The listing builds one solid part. Answer for the finished solid, in the listing's coordinates (mm). A direction names the side the tool comes from. Round coordinates to 2 decimals unless told otherwise and drop trailing zeros. Loops run counter-clockwise (first coordinate to the right, second up) from the corner with the lowest first, then second, coordinate; pieces in that order, holes last. Notation, with made-up numbers: M -38,76 L -12,76 A21 cw -12,82 Z; hole C 69,-5 d6. An arc over 180 degrees is marked long. Answer as a JSON object with one key per item and string values.
```python
from build123d import *

# Parameters (mm, degrees)
F0_W      = 380
F0_H      = 180
F1_DEPTH  = 10
F2_W      = 6
F2_H      = 180
F3_DEPTH  = 2
F5_DEPTH  = 5.6
F7_DEPTH  = 5.8
F8_R      = 3.5
F9_DEPTH  = 5
F9_TAPER  = 1
F10_R     = 3.5
F11_DEPTH = 5


with BuildPart() as f1:
    # F0 (on Top) → F1 (new body)
    with BuildSketch(Plane.XY):
        Rectangle(F0_W, F0_H)
    extrude(amount=F1_DEPTH)

    # F2 (on face) → F3 (join)
    with BuildSketch(Plane.XY.offset(10)):
        Rectangle(F2_W, F2_H)
    extrude(amount=F3_DEPTH)

    # F4 (on face) → F5 (cut)
    with BuildSketch(Plane.XY.offset(10)):
        with BuildLine():
            ThreePointArc((-4.5, 49), (-6.2573593129, 53.2426406871), (-10.5, 55))
            Line((-10.5, 55), (-139.5, 55))
            ThreePointArc((-139.5, 55), (-143.7426406871, 53.2426406871), (-145.5, 49))
            Line((-145.5, 49), (-145.5, -49))
            ThreePointArc((-145.5, -49), (-143.7426406871, -53.2426406871), (-139.5, -55))
            Line((-139.5, -55), (-10.5, -55))
            ThreePointArc((-10.5, -55), (-6.2573593129, -53.2426406871), (-4.5, -49))
            Line((-4.5, -49), (-4.5, 49))
        make_face()
    extrude(amount=-F5_DEPTH, mode=Mode.SUBTRACT)

    # F6 (on face) → F7 (join)
    with BuildSketch(Plane.XY.offset(10)):
        with BuildLine():
            Line((140.3, 55.4), (10.5, 55.4))
            ThreePointArc((10.5, 55.4), (6.2573593129, 53.6426406871), (4.5, 49.4))
            Line((4.5, 49.4), (4.5, -49.4))
            ThreePointArc((4.5, -49.4), (6.2573593129, -53.6426406871), (10.5, -55.4))
            Line((10.5, -55.4), (140.3, -55.4))
            ThreePointArc((140.3, -55.4), (144.5426406871, -53.6426406871), (146.3, -49.4))
            Line((146.3, -49.4), (146.3, 49.4))
            ThreePointArc((146.3, 49.4), (144.5426406871, 53.6426406871), (140.3, 55.4))
        make_face()
    extrude(amount=F7_DEPTH)

    # F8 (on face) → F9 (join)
    with BuildSketch(Plane.XY.offset(10)):
        with Locations((-156.5, 44)):
            Circle(F8_R)
        with Locations((-156.5, -44)):
            Circle(F8_R)
    extrude(amount=F9_DEPTH, taper=F9_TAPER)

    # F10 (on face) → F11 (cut)
    with BuildSketch(Plane.XY.offset(10)):
        with Locations((157.3, 44.4)):
            Circle(F10_R)
        with Locations((157.3, -44.4)):
            Circle(F10_R)
    extrude(amount=-F11_DEPTH, mode=Mode.SUBTRACT)


solid = f1.part
```
Item 1: The part is cut by section C-C (y = 63). Give the vertices of the cut face in (x, z).
Values follow:
{"outline": "M -190,0 L 190,0 L 190,10 L 3,10 L 3,12 L -3,12 L -3,10 L -190,10 Z"}
Item 2: Which of the six approach directions +Z, -Z, +X, -X, +Y, -Y give full straight-line access (tool end or side, diameter ignored) to faces 1 (the face through (-153.308, 42.676, 12.535)), 2 (the face through (-3, 90, 6)), 3 (the face through (-157, -44, 15))?
Values follow:
{"face 1": "+Z", "face 2": "+Z, -Z, +X, -X, +Y", "face 3": "+Z, -X, +Y, -Y"}
Item 3: Flat-ended cylindrical pins translate along their axes: P1, Ø1, axis at y = 53.5, z = 12.5, coming from the +X side; P2, Ø3, axis at x = 6.5, z = 12, coming from the +Y side; P3, Ø3.5, axis at x = -155, y = -42.5, coming from the +Z side; P4, Ø4, axis at x = 157.3, y = -44.4, coming from the -Z side. Find the tip coordinate at first contact, or state that the pin passes through.
Values follow:
{"P1": "x = 145.1", "P2": "y = 54.85", "P3": "z = 15", "P4": "z = 0"}
Item 4: The part is cut by section D-D (x = 157.3). Give the vertices of the cut face in (y, z).
Values follow:
{"outline": "M -90,0 L 90,0 L 90,10 L 47.9,10 L 47.9,5 L 40.9,5 L 40.9,10 L -40.9,10 L -40.9,5 L -47.9,5 L -47.9,10 L -90,10 Z"}
Item 5: The part is cut by section A-A (y = -32.5). Give the vertices of the cut face in (x, z).
Values follow:
{"outline": "M -190,0 L 190,0 L 190,10 L 146.3,10 L 146.3,15.8 L 4.5,15.8 L 4.5,10 L 3,10 L 3,12 L -3,12 L -3,10 L -4.5,10 L -4.5,4.4 L -145.5,4.4 L -145.5,10 L -190,10 Z"}
Item 6: The part is cut by section B-B (x = -94). Give the vertices of the cut face in (y, z).
Values follow:
{"outline": "M -90,0 L 90,0 L 90,10 L 55,10 L 55,4.4 L -55,4.4 L -55,10 L -90,10 Z"}
Item 7: Straight lines are drawn through the part: line 1 (Y direction, x = 157.3, z = 6.25); line 2 (X direction, y = -16, z = 4.5); line 3 (X direction, y = -20, z = 11). For each, find the intervals that lie inside material, in ascending order.
Values follow:
{"line 1": "-90 to -47.9, -40.9 to 40.9, 47.9 to 90", "line 2": "-190 to -145.5, -4.5 to 190", "line 3": "-3 to 3, 4.5 to 146.3"}
Item 8: Determine the mould class of faces 4 (the face through (153.803, 44.554, 7.535)), 5 (the face through (-190, -1, 5)), 6 (the face through (74, 1, 15.8)), 7 (the face through (157, 44, 5)) for opening direction X: released by +X, released by -X, zero draft, split by the parting line, or undercut.
Values follow:
{"face 4": "undercut", "face 5": "released by -X", "face 6": "zero draft", "face 7": "undercut"}
